Source: CAD feature listing. Evaluate the final solid. Frame: model axes, mm. Face numbers are marked on the shaded views. A direction names the side the tool comes from. Give positions to 0.01 mm unless a question says otherwise; leave off trailing zeros. Loops run counter-clockwise (first coordinate to the right, second up) from the corner with the lowest first, then second, coordinate; pieces in that order, holes last. Notation, with made-up numbers: (0.25, 29) - (47.25, 29) arc R28 cw to (47.25, 63) - close; hole circle Ø3 at (25, -13). An arc over 180 degrees is marked (long way). Write each question's results on one line, items separated by ' | '. Start each with the question number.
(1) Cut plane B-B on x = -1.75. Return the cut outline in (y, z).
(2) Contact query for flat-ended pins moving along their axis: pin 1 (5 mm diameter, centred on x = 1.5, y = 16, fed in from +Z); pin 2 (3 mm diameter, centred on x = -2.5, z = 13, fed in from +Y); pin 3 (1.5 mm diameter, centred on y = 15.5, z = 16.5, fed in from -X). Output: stop coordinate, or through.
(3) Cut plane D-D on y = 7. Return the cut outline in (x, z).
(4) Reachability of the marked faces 1, 2 and 3 from +Z, -Z, +X, -X, +Y, -Y: full face, straight path, thin tool, end or side. Return the list, or none.
(5) Material intervals for line 1 along X through (y, z) = (15, 18.25); line 2 along Y through (x, z) = (-7.75, 14); line 3 along X through (y, z) = (15.75, 3), sorted ascending. Write a range as [from, to].
(6) Cut plane C-C on z = 12.5. Return the cut outline in (x, y).
(7) Cut plane A-A on y = 18.5. Return the cut outline in (x, z).
from build123d import *

# Parameters (mm, degrees)
BOSS_EXTRUDE2_DEPTH = 20
SKETCH3_W           = 5
SKETCH3_H           = 20
BOSS_EXTRUDE4_DEPTH = 5
CUT_EXTRUDE1_DEPTH  = 5
SKETCH5_W           = 5
SKETCH5_H           = 20
BOSS_EXTRUDE5_DEPTH = 5
CUT_EXTRUDE2_DEPTH  = 5
SKETCH7_W           = 5
SKETCH7_H           = 15
BOSS_EXTRUDE6_DEPTH = 5
BOSS_EXTRUDE7_DEPTH = 20
CUT_EXTRUDE3_DEPTH  = 20
BOSS_EXTRUDE8_DEPTH = 5
BOSS_EXTRUDE9_DEPTH = 5


with BuildPart() as part:
    # Sketch2 → Boss-Extrude2 (new body)
    with BuildSketch(Plane(origin=(0, 0, 0), x_dir=(1, 0, 0), z_dir=(0, 1, 0))):
        Polygon((0, 0), (10, 0), (10, -15), (5, -15), (-5, -5), (0, -5), align=None)
    extrude(amount=BOSS_EXTRUDE2_DEPTH)

    # Sketch3 → Boss-Extrude4 (add)
    with BuildSketch(Plane.XY.offset(15)):
        with Locations((7.5, 10)):
            Rectangle(SKETCH3_W, SKETCH3_H)
    extrude(amount=BOSS_EXTRUDE4_DEPTH)

    # Sketch4 → Cut-Extrude1 (cut)
    with BuildSketch(Plane.ZY.offset(-5)):
        Polygon((15, 20), (20, 15), (20, 20), align=None)
    extrude(amount=-CUT_EXTRUDE1_DEPTH, mode=Mode.SUBTRACT)

    # Sketch5 → Boss-Extrude5 (add)
    with BuildSketch(Plane.ZY):
        with Locations((2.5, 10)):
            Rectangle(SKETCH5_W, SKETCH5_H)
    extrude(amount=BOSS_EXTRUDE5_DEPTH)

    # Sketch6 → Cut-Extrude2 (cut)
    with BuildSketch(Plane(origin=(0, 0, 0), x_dir=(-1, 0, 0), z_dir=(0, 0, -1))):
        Polygon((0, 20), (5, 20), (5, 15), align=None)
    extrude(amount=-CUT_EXTRUDE2_DEPTH, mode=Mode.SUBTRACT)

    # Sketch7 → Boss-Extrude6 (add)
    with BuildSketch(Plane.ZY.offset(5)):
        with Locations((2.5, 7.5)):
            Rectangle(SKETCH7_W, SKETCH7_H)
    extrude(amount=BOSS_EXTRUDE6_DEPTH)

    # Sketch8 → Boss-Extrude7 (add)
    with BuildSketch(Plane(origin=(0, 0, 0), x_dir=(-1, 0, 0), z_dir=(0, -1, 0))):
        Polygon((10, -5), (5, -5), (-5, -15), (5, -15), (10, -10), align=None)
    extrude(amount=-BOSS_EXTRUDE7_DEPTH)

    # 3DSketch1 → Cut-Extrude3 (cut, along a direction that is not the sketch's normal)
    with BuildSketch(Plane(origin=(-5, 10, 15), x_dir=(0.7071067811865476, 0.7071067811865476, 0), z_dir=(-0.5773502691896257, 0.5773502691896257, 0.577350269189626))):
        Polygon((0, 0), (14.142135624, 0), (7.071067812, 12.247448714), (0, 12.247448714), (-3.535533906, 6.123724357), align=None)
    extrude(amount=CUT_EXTRUDE3_DEPTH, dir=(0, 1, 0), mode=Mode.SUBTRACT)

    # Sketch9 → Boss-Extrude8 (add)
    with BuildSketch(Plane(origin=(0, 0, 0), x_dir=(-1, 0, 0), z_dir=(0, -1, 0))):
        Polygon((5, -20), (10, -15), (10, -10), (5, -15), (-5, -15), (-5, -20), align=None)
    extrude(amount=-BOSS_EXTRUDE8_DEPTH)

    # Sketch10 → Boss-Extrude9 (add)
    with BuildSketch(Plane(origin=(0, 5, 0), x_dir=(1, 0, 0), z_dir=(0, 1, 0))):
        Polygon((0, -15), (5, -20), (5, -15), align=None)
    extrude(amount=BOSS_EXTRUDE9_DEPTH)


solid = part.part
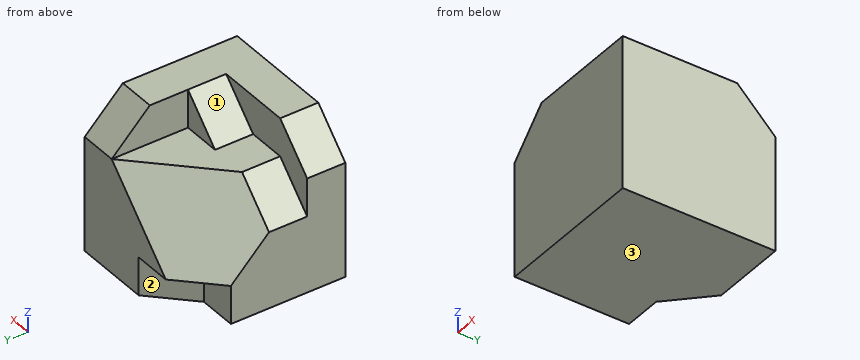
Ans:
1) outline: (0, 0) - (18.25, 0) - (18.25, 5) - (20, 5) - (20, 8.25) - (13.25, 15) - (5, 15) - (5, 20) - (0, 20) - close
2) pin 1: z = 15 | pin 2: y = 16.62 | pin 3: x = 5
3) outline: (-10, 0) - (10, 0) - (10, 20) - (5, 20) - (0, 15) - (-5, 15) - (-10, 10) - close
4) face 1: +Z, -X, +Y | face 2: -Z, -X, +Y | face 3: -Z, +X, -X, +Y, -Y
5) line 1: [5, 10] | line 2: [0, 5] | line 3: [-4.25, 10]
6) outline: (-10, 0) - (10, 0) - (10, 20) - (2.5, 20) - (-7.5, 10) - (-7.5, 5) - (-10, 5) - close
7) outline: (-6.5, 5) - (-1.5, 5) - (-1.5, 0) - (10, 0) - (10, 16.5) - (5, 16.5) - (5, 15) - (3.5, 15) - close
